Geometry check sheet. Reference: the model listing, model coordinates, mm. A direction names the side the tool comes from. Give positions to 0.01 mm unless a question says otherwise; leave off trailing zeros. Loops run counter-clockwise (first coordinate to the right, second up) from the corner with the lowest first, then second, coordinate; pieces in that order, holes last.
1. Tool access check on faces 1 (the cylindrical face through (42.54, 1.57, 23.59)), 2 (the flat face through (4.7, 3.175, 15.3)), 3 (the flat face through (34.925, 8, 13)). Record the directions out of +Z, -Z, +X, -X, +Y, -Y that give a thin tool (end or side, any length) a straight path to the whole face; none if there is none.
2. Release check for a two-part mould opening along Z. For faces 4 (the flat face through (22, 6, 25.4)), 5 (the cylindrical face through (37.647, 1.565, 13.761)), 6 (the flat face through (39.6, 3.175, 15.3)) record: +Z half, -Z half, draft (parallel to the pull), parting line (faces both ways), or undercut.
3. Cross-section at D-D, the plane y = 5. Record the cut outline in (x, z) (3 decimals), plus the area to 3 significant figures.
4. Go/stop test with flat-tipped pins: pin 1 Ø6 at (y, z) = (9.5, 14) entering from -X (3 decimals); pin 2 Ø3 at (x, z) = (39, 8.5) entering from +Y (3 decimals); pin 3 Ø1 at (x, y) = (8, 8.5) entering from -Z; pin 4 Ø7.5 at (y, z) = (7, 11) entering from +X (3 decimals). Record where each tip stops, or that it passes through.
5. Material ranges on L1, parallel to X at y = 1.2, z = 12.7; L2, parallel to X at y = 9.75, z = 8.25 (3 decimals); L3, parallel to Y at x = 36, z = 2 (3 decimals), recorded low to high.
6. Cross-section at C-C, the plane z = 9. Record the cut outline in (x, y) (3 decimals), plus the area to 3 significant figures.
7. Cross-section at A-A, the plane z = 12.7. State how many separate pieces and enclosed holes the cut face has, plus the area to 3 significant figures.
8. Cross-section at B-B, the plane x = 4. Record the cut outline in (y, z) (3 decimals), plus the area to 3 significant figures.
from build123d import *

# Parameters (mm, degrees)
BOSS_EXTRUDE1_DEPTH     = 25.4
CUT_EXTRUDE1_DEPTH      = 53.073871807
CUT_EXTRUDE1_DEPTH_BACK = 53.073871807
SKETCH2_R               = 2.3
FILLET1_R               = 6.35


with BuildPart() as part:
    # Sketch1 → Boss-Extrude1 (new body)
    with BuildSketch(Plane.XY):
        Polygon((0, 0), (0, 3.175), (9.525, 3.175), (9.525, 12.7), (34.925, 12.7), (34.925, 3.175), (44.45, 3.175), (44.45, 0), align=None)
    extrude(amount=BOSS_EXTRUDE1_DEPTH)

    # Sketch2 → Cut-Extrude1 (cut, two sides: drawn at the far end of the back side and taken through both)
    with BuildSketch(Plane(origin=(0, 3.175, 0), x_dir=(1, 0, 0), z_dir=(0, 1, 0)).offset(-CUT_EXTRUDE1_DEPTH_BACK)):
        with Locations(Location((4.7625, -12.7, 0), (0, 0, 270))):
            Circle(SKETCH2_R)
        with Locations(Location((39.6875, -12.7, 0), (0, 0, 270))):
            Circle(SKETCH2_R)
    extrude(amount=CUT_EXTRUDE1_DEPTH + CUT_EXTRUDE1_DEPTH_BACK, mode=Mode.SUBTRACT)

    # Fillet1
    fillet1_edges = [part.edges().sort_by_distance(p)[0] for p in [
        (44.45, 1.5875, 0),
        (0, 1.5875, 25.4),
        (0, 1.5875, 0),
        (44.45, 1.5875, 25.4),
    ]]
    fillet(fillet1_edges, radius=FILLET1_R)


solid = part.part
Result:
1. face 1: +Z, +X, +Y, -Y
1. face 2: +Z, -Z, -X, +Y
1. face 3: +Z, -Z, +X, +Y
2. face 4: +Z half
2. face 5: undercut
2. face 6: draft
3. outline: (9.525, 0) - (34.925, 0) - (34.925, 25.4) - (9.525, 25.4) - close
3. area: 645 mm2
4. pin 1: stops at x = 9.525
4. pin 2: stops at y = 3.175
4. pin 3: passes through
4. pin 4: stops at x = 34.925
5. L1: x = 0 to 2.46, 7.06 to 37.39, 41.99 to 44.45
5. L2: x = 9.525 to 34.925
5. L3: y = 0 to 3.175
6. outline: (0, 0) - (44.45, 0) - (44.45, 3.175) - (34.925, 3.175) - (34.925, 12.7) - (9.525, 12.7) - (9.525, 3.175) - (0, 3.175) - close
6. area: 383 mm2
7. separate pieces: 3
7. enclosed holes: 0
7. area: 354 mm2
8. outline: (0, 0.451) - (3.175, 0.451) - (3.175, 10.53) - (0, 10.53) - close; (0, 14.87) - (3.175, 14.87) - (3.175, 24.949) - (0, 24.949) - close
8. area: 64.0 mm2
